Model file for the job. Use its own axes, mm. A direction names the side the tool comes from. Coordinates: 2 decimals unless noted, no trailing zeros. Loops run counter-clockwise (first coordinate to the right, second up) from the corner with the lowest first, then second, coordinate; pieces in that order, holes last. Notation, with made-up numbers: M 5.25,3 L 16.25,3 A29 cw 16.25,41 Z; hole C 47.25,86.5 d2. An arc over 180 degrees is marked long. Write item = value, one per line. Start each with the question number.
from build123d import *

# Parameters (mm, degrees)
SKETCH1_W               = 160
SKETCH1_H               = 129
BOSS_EXTRUDE1_DEPTH     = 8
SKETCH1_3_R             = 4
CUT_EXTRUDE2_DEPTH      = 104.074002542
FILLET1_R               = 10
CUT_EXTRUDE4_DEPTH      = 1
CUT_EXTRUDE4_DEPTH_BACK = 3
CUT_EXTRUDE4_START      = 8
CUT_EXTRUDE9_DEPTH      = 104.074002542
CUT_EXTRUDE10_START     = 8
SKETCH1_17_R            = 2.5
SKETCH1_17_R_2          = 10
CUT_EXTRUDE10_DEPTH     = 5
BOSS_EXTRUDE4_START     = 10
BOSS_EXTRUDE4_DEPTH     = 10
FILLET2_R               = 10


with BuildPart() as part:
    # Sketch1 → Boss-Extrude1 (new body)
    with BuildSketch(Plane(origin=(0, 0, 0), x_dir=(1, 0, 0), z_dir=(0, 1, 0))):
        Rectangle(SKETCH1_W, SKETCH1_H)
    extrude(amount=BOSS_EXTRUDE1_DEPTH)

    # Sketch1<3> → Cut-Extrude2 (cut, through all)
    with BuildSketch(Plane(origin=(0, 0, 0), x_dir=(1, 0, 0), z_dir=(0, 1, 0))):
        with Locations(Location((-70, 54.5, 0), (0, 0, 270))):
            Circle(SKETCH1_3_R)
        with Locations(Location((-70, -54.5, 0), (0, 0, 270))):
            Circle(SKETCH1_3_R)
        with Locations(Location((70, -54.5, 0), (0, 0, 90))):
            Circle(SKETCH1_3_R)
        with Locations(Location((70, 54.5, 0), (0, 0, 90))):
            Circle(SKETCH1_3_R)
    extrude(amount=CUT_EXTRUDE2_DEPTH, mode=Mode.SUBTRACT)

    # Fillet1
    fillet1_edges = [part.edges().sort_by_distance(p)[0] for p in [
        (80, 4, 64.5),
        (-80, 4, 64.5),
        (-80, 4, -64.5),
        (80, 4, -64.5),
    ]]
    fillet(fillet1_edges, radius=FILLET1_R)

    # Sketch1<11> → Cut-Extrude4 (cut, two sides: drawn at the far end of the back side and taken through both)
    with BuildSketch(Plane(origin=(0, 0, 0), x_dir=(1, 0, 0), z_dir=(0, 1, 0)).offset(CUT_EXTRUDE4_START - CUT_EXTRUDE4_DEPTH_BACK)):
        with BuildLine():
            Line((53, -40), (-53, -40))
            ThreePointArc((-53, -40), (-57.949747468, -37.949747468), (-60, -33))
            Line((-60, -33), (-60, 33))
            ThreePointArc((-60, 33), (-57.949747468, 37.949747468), (-53, 40))
            Line((-53, 40), (53, 40))
            ThreePointArc((53, 40), (57.949747468, 37.949747468), (60, 33))
            Line((60, 33), (60, -33))
            ThreePointArc((60, -33), (57.949747468, -37.949747468), (53, -40))
        make_face()
    extrude(amount=CUT_EXTRUDE4_DEPTH + CUT_EXTRUDE4_DEPTH_BACK, mode=Mode.SUBTRACT)

    # Sketch1<13> → Cut-Extrude9 (cut, through all)
    with BuildSketch(Plane(origin=(0, 0, 0), x_dir=(1, 0, 0), z_dir=(0, 1, 0))):
        with BuildLine():
            Line((-70, -64.5), (70, -64.5))
            ThreePointArc((70, -64.5), (65.25658351, -63.303408431), (61.648353456, -60))
            Line((61.648353456, -60), (-61.648353456, -60))
            ThreePointArc((-61.648353456, -60), (-65.25658351, -63.303408431), (-70, -64.5))
        make_face()
        with BuildLine():
            ThreePointArc((61.648353456, 60), (65.25658351, 63.303408431), (70, 64.5))
            Line((70, 64.5), (-69.999999984, 64.5))
            ThreePointArc((-69.999999984, 64.5), (-65.256583502, 63.303408427), (-61.648353456, 60))
            Line((-61.648353456, 60), (61.648353456, 60))
        make_face()
    extrude(amount=CUT_EXTRUDE9_DEPTH, mode=Mode.SUBTRACT)

    # Sketch1<17> → Cut-Extrude10 (cut)
    with BuildSketch(Plane(origin=(0, 0, 0), x_dir=(1, 0, 0), z_dir=(0, 1, 0)).offset(CUT_EXTRUDE10_START)):
        with Locations(Location((0, 31.25, 0), (0, 0, 270))):
            Circle(SKETCH1_17_R)
        with Locations((-70, 54.5)):
            Circle(SKETCH1_17_R_2)
        with Locations((70, 54.5)):
            Circle(SKETCH1_17_R_2)
        with Locations((-70, -54.5)):
            Circle(SKETCH1_17_R_2)
        with Locations((70, -54.5)):
            Circle(SKETCH1_17_R_2)
        with Locations(Location((0, -32.75, 0), (0, 0, 270))):
            Circle(SKETCH1_17_R)
    extrude(amount=-CUT_EXTRUDE10_DEPTH, mode=Mode.SUBTRACT)

    # Sketch1<18> → Boss-Extrude4 (add)
    with BuildSketch(Plane(origin=(0, 0, 0), x_dir=(1, 0, 0), z_dir=(0, 1, 0)).offset(BOSS_EXTRUDE4_START)):
        with BuildLine():
            ThreePointArc((60.460607986, 57.5), (60.967568701, 58.791291743), (61.648353456, 60))
            Line((61.648353456, 60), (-61.648353456, 60))
            ThreePointArc((-61.648353456, 60), (-60.967568701, 58.791291743), (-60.460607986, 57.5))
            Line((-60.460607986, 57.5), (60.460607986, 57.5))
        make_face()
        with BuildLine():
            Line((-80, 54.500000177), (-80, -54.5))
            ThreePointArc((-80, -54.5), (-79.354143467, -50.964466094), (-77.5, -47.885621722))
            Line((-77.5, -47.885621722), (-77.5, 47.885621722))
            ThreePointArc((-77.5, 47.885621722), (-79.354143498, 50.964466177), (-80, 54.500000177))
        make_face()
        with BuildLine():
            ThreePointArc((77.5, -47.885621722), (79.354143467, -50.964466094), (80, -54.5))
            Line((80, -54.5), (80, 54.5))
            ThreePointArc((80, 54.5), (79.354143467, 50.964466094), (77.5, 47.885621722))
            Line((77.5, 47.885621722), (77.5, -47.885621722))
        make_face()
        with BuildLine():
            Line((-61.648353456, -60), (61.648353456, -60))
            ThreePointArc((61.648353456, -60), (60.967568701, -58.791291743), (60.460607986, -57.5))
            Line((60.460607986, -57.5), (-60.460607986, -57.5))
            ThreePointArc((-60.460607986, -57.5), (-60.967568701, -58.791291743), (-61.648353456, -60))
        make_face()
    extrude(amount=-BOSS_EXTRUDE4_DEPTH)

    # Fillet2
    # the kernel refuses this fillet: 10 mm, written as the material it adds along each edge
    with BuildSketch(Plane(origin=(61.648353456, 0, 60), x_dir=(0.6702455950029323, 0, 0.7421393685684416), z_dir=(0, 1, 0)), Plane(origin=(-61.648353456, 0, -60), x_dir=(-0.6702455950029282, 0, -0.7421393685684453), z_dir=(0, 1, 0))) as fillet2_piece_1:
        with BuildLine():
            CenterArc((4.547663341, -9.884436465), FILLET2_R, 98.719009802, 39.194967426)
            Line((-2.873730345, -3.181980515), (0, 0))
            ThreePointArc((0, 0), (1.51588778, -0.115563535), (3.03177556, 0))
        make_face()
    extrude(amount=3)
    with BuildSketch(Plane(origin=(-61.648353456, 0, 60), x_dir=(1, 0, 0), z_dir=(0, 1, 0))) as fillet2_piece_2:
        with BuildLine():
            CenterArc((4.287578116, -10), FILLET2_R, 90, 39.194967426)
            ThreePointArc((-2.032034214, -2.25), (-0.930252859, -1.20245595), (0, 0))
            Line((0, 0), (4.287578116, 0))
        make_face()
    extrude(amount=3)
    with BuildSketch(Plane(origin=(61.648353456, 0, -60), x_dir=(0.6702455950029361, 0, -0.7421393685684381), z_dir=(0, 1, 0))) as fillet2_piece_3:
        with BuildLine():
            CenterArc((4.547663341, 9.884436465), FILLET2_R, 222.086022772, 39.194967426)
            Line((-2.873730345, 3.181980515), (0, 0))
            ThreePointArc((0, 0), (1.51588778, 0.115563535), (3.03177556, 0))
        make_face()
    extrude(amount=3)


solid = part.part
Item 1: Cut at C-C (x = 0). Give the cut face in (y, z).
Item 2: Pull direction Z, two halves, no side cores. Call faces 3 (the cylindrical face through (-73.549, 1.479, 56.346)), 4 (the flat face through (0, 0, -2)), 5 (the flat face through (-1, 5, -60)): +Z half, -Z half, draft (parallel to the pull), parting line (faces both ways), or undercut.
Item 3: Pin check, flat tips, straight feed: pin 1 Ø1 at (x, y) = (-13.5, 9.5) entering from +Z; pin 2 Ø1.5 at (x, z) = (-1, -30) entering from +Y; pin 3 Ø4 at (x, y) = (-39.5, 1.5) entering from -Z. Stop position of each tip, or through.
Item 4: Cut at B-B (x = 34.5). Give the cut face in (y, z).
Item 5: Probe L1, parallel to X at y = 1.2, z = 54.5; L2, parallel to Z at x = 37, y = 6.5; L3, parallel to Z at x = 57, y = 8.25. List the from-to ranges inside material, lowest first.
Item 6: Cut at A-A (z = -19). Give the cut face in (x, y), plus the area to 3 significant figures.
Item 7: 3-axis set-ups, long thin cutter, end or side, ignore diameter. For faces 1 (the cylindrical face through (73.549, 1.479, -56.346)), 2 (the cylindrical face through (58, 6.5, 37.9)): which of +Z, -Z, +X, -X, +Y, -Y reach the whole face in a straight line?
Reported:
q1.outline = M 0,-60 L 10,-60 L 10,-57.5 L 8,-57.5 L 8,-40 L 5,-40 L 5,-33.75 L 3,-33.75 L 3,-28.75 L 5,-28.75 L 5,30.25 L 3,30.25 L 3,35.25 L 5,35.25 L 5,40 L 8,40 L 8,57.5 L 10,57.5 L 10,60 L 0,60 Z
q2.face_3 = undercut
q2.face_4 = draft
q2.face_5 = -Z half
q3.pin_1 = 60
q3.pin_2 = 3
q3.pin_3 = -60
q4.outline = M 0,-60 L 10,-60 L 10,-57.5 L 8,-57.5 L 8,-40 L 5,-40 L 5,40 L 8,40 L 8,57.5 L 10,57.5 L 10,60 L 0,60 Z
q5.L1 = -80 to -74, -66 to 66, 74 to 80
q5.L2 = -60 to -40, 40 to 60
q5.L3 = -60 to -57.5, 57.5 to 60
q6.outline = M -80,0 L 80,0 L 80,10 L 77.5,10 L 77.5,8 L 60,8 L 60,5 L -60,5 L -60,8 L -77.5,8 L -77.5,10 L -80,10 Z
q6.area = 930 mm^2
q7.face_1 = +Y, -Y
q7.face_2 = +Y
